from build123d import *

# Parameters (mm, degrees)
F4_DEPTH = 5
F3_R     = 10.75
F5_DEPTH = 1.3
F6_R     = 1
F7_DEPTH = 22.1
F8_R     = 1


with BuildPart() as f2:
    # F0 (on Front) → F2 (revolve)
    with BuildSketch(Plane.XZ):
        with BuildLine():
            ThreePointArc((-10.5, 0), (-7.4246212025, 7.4246212025), (0, 10.5))
            Line((0, 10.5), (0, 12.5))
            ThreePointArc((0, 12.5), (-8.8388347648, 8.8388347648), (-12.5, 0))
            Line((-12.5, 0), (-10.5, 0))
        make_face()
    revolve(axis=Axis((0, 0, 21.9115), (0, 0, 1)))

    # F4 (add): a face of the model
    f4_faces = [f2.faces().sort_by_distance(p)[0] for p in [
        (12.1464466094, 0, 0),
    ]]
    extrude(f4_faces, amount=F4_DEPTH)

    # F3 (on Top) → F5 (cut)
    with BuildSketch(Plane.XY):
        Circle(F3_R)
    extrude(amount=-F5_DEPTH, mode=Mode.SUBTRACT)

    # F6 (on Top) → F7 (cut)
    with BuildSketch(Plane.XY):
        Circle(F6_R)
    extrude(amount=F7_DEPTH, mode=Mode.SUBTRACT)

    # F8
    f8_edges = [f2.edges().sort_by_distance(p)[0] for p in [
        (10.5, 0, -5),
        (0, -1, 10.452272),
        (0, 1, 10.452272),
    ]]
    fillet(f8_edges, radius=F8_R)


solid = f2.part
Model file for the job. Use its own axes, mm. Give positions to 0.01 mm unless a question says otherwise; leave off trailing zeros. Order: outer loops, then holes, each group sorted by start corner. A loop starts at its lowest first (then second) coordinate and runs counter-clockwise, first axis right, second up. Notation, with made-up numbers: (74.25, 70) - (78.25, 70) arc R19 ccw to (78.25, 90) - close; hole circle Ø8 at (-31, -24.75). An arc over 180 degrees is marked (long way). Write item = value, one per line. Start each with the question number.
1. Drop flat-ended pins along their axis: P1, Ø6, axis at x = -1.5, y = 6, coming from the +Z side; P2, Ø3, axis at y = 9.5, z = 5.5, coming from the +X side; P3, Ø3, axis at x = 2, z = 10, coming from the -Y side. Give the stop position or say it passes through.
2. Probe line 1 along Y through (x, z) = (0, -2.95); line 2 along Y through (x, z) = (0, -0.65). List the from-to ranges inside material, lowest first.
3. Cut at A-A, the plane z = 1.5. List the corners of the cut face in (x, y), and give its area (3 significant figures).
4. Two-plate mould, pull along Y, no slides. Class faces 1 (the cylindrical face through (-11.923, -3.755, -2.465)), 2 (the cylindrical face through (-1.4, 10.66, -0.64)), 3 (the flat face through (-11, 4, -5)), 4 (the cylindrical face through (1, 0, 12)): pulls with the +Y half, pulls with the -Y half, needs draft (parallel to the pull), parting line crosses it, or undercut.
Taken from the geometry:
q1.P1 = 12.09
q1.P2 = 8.15
q1.P3 = -8.98
q2.line_1 = -12.5 to -10.5, 10.5 to 12.5
q2.line_2 = -12.5 to -10.75, 10.75 to 12.5
q3.outline = circle Ø24.82 at (0, 0); hole circle Ø20.78 at (0, 0)
q3.area = 145 mm²
q4.face_1 = parting line crosses it
q4.face_2 = undercut
q4.face_3 = needs draft
q4.face_4 = undercut
